Could you check a few things on this model? Use its own coordinates, in mm. A direction names the side the tool comes from. Round coordinates to 2 decimals unless told otherwise and drop trailing zeros. Loops run counter-clockwise (first coordinate to the right, second up) from the corner with the lowest first, then second, coordinate; pieces in that order, holes last. Notation, with made-up numbers: (-6, -32) -> (18, -32) arc R8 ccw to (18, -20) -> close; hole circle Ø2 at (22.25, 80). An arc over 180 degrees is marked (long way). Write each question's results on one line, items separated by ' | '.
from build123d import *

# Parameters (mm, degrees)
F0_R     = 38.1
F1_DEPTH = 127
F2_T     = -4
F3_R     = 38.1
F3_R_2   = 35.5
F4_DEPTH = 15
F5_R     = 3


with BuildPart() as f1:
    # F0 (on Top) → F1 (new body)
    with BuildSketch(Plane.XY):
        Circle(F0_R)
    extrude(amount=F1_DEPTH)

    # F2
    f2_openings = [f1.faces().sort_by_distance(p)[0] for p in [
        (0, 0, 127),
    ]]
    offset(amount=F2_T, openings=f2_openings)

    # F3 (on face) → F4 (cut)
    with BuildSketch(Plane.XY.offset(127)):
        Circle(F3_R)
        Circle(F3_R_2, mode=Mode.SUBTRACT)
    extrude(amount=-F4_DEPTH, mode=Mode.SUBTRACT)

    # F5
    f5_edges = [f1.edges().sort_by_distance(p)[0] for p in [
        (-38.1, 0, 0),
        (-34.1, 0, 4),
    ]]
    fillet(f5_edges, radius=F5_R)


solid = f1.part
1) I'm going to push flat-ended pins straight in: pin 1 (2 mm diameter, centred on y = 13, z = 34, fed in from -X); pin 2 (3 mm diameter, centred on y = 20, z = 99.5, fed in from -X); pin 3 (1.5 mm diameter, centred on x = 4.5, z = 51.5, fed in from -Y) (3 decimals). Where does each tip first touch, or does it pass through?
Model answer:
pin 1: stops at x = -36.16 | pin 2: stops at x = -33.31 | pin 3: stops at y = -37.915
2) I need wall thicknesses on line 1 (Y direction, x = 0, z = 102); line 2 (Y direction, x = 29, z = 46.5); line 3 (X direction, y = 15.5, z = 40). Which ranges of each line are inside material? Lowest first, please.
Model answer:
line 1: y = -38.1 to -34.1, 34.1 to 38.1 | line 2: y = -24.71 to -17.94, 17.94 to 24.71 | line 3: x = -34.8 to -30.37, 30.37 to 34.8
3) I want a section at A-A, the plane z = 98.5. Write out the boundary of the cut face in (x, y), plus the area to 3 significant figures.
Model answer:
outline: circle Ø76.2 at (0, 0); hole circle Ø68.2 at (0, 0) | area: 907 mm2
4) I want a section at B-B, the plane y = 0. Write out the boundary of the cut face in (x, z), plus the area to 3 significant figures.
Model answer:
outline: (-38.1, 3) arc R3 ccw to (-35.1, 0) -> (35.1, 0) arc R3 ccw to (38.1, 3) -> (38.1, 112) -> (35.5, 112) -> (35.5, 127) -> (34.1, 127) -> (34.1, 7) arc R3 cw to (31.1, 4) -> (-31.1, 4) arc R3 cw to (-34.1, 7) -> (-34.1, 127) -> (-35.5, 127) -> (-35.5, 112) -> (-38.1, 112) -> close | area: 1,210 mm2
5) If we mould it in two halves opening along X, with no side actions, what happens to faces 1 (the flat face through (34, 11, 112)), 2 (the cylindrical face through (-30.235, -23.183, 56.737)), 3 (the flat face through (0, 0, 4)), 4 (the cylindrical face through (-4.44, 33.81, 66.16))? For each: released by +X, released by -X, zero draft, split by the parting line, or undercut.
Model answer:
face 1: zero draft | face 2: split by the parting line | face 3: undercut | face 4: undercut
6) For faces 5 (the cylindrical face through (-7.696, -34.656, 119.605)), 6 (the flat face through (-32, 13, 127)), which set-ups out of +Z, -Z, +X, -X, +Y, -Y let a thin tool reach every point of the face, with its end or its side?
Model answer:
face 5: +Z | face 6: +Z, +X, -X, +Y, -Y
